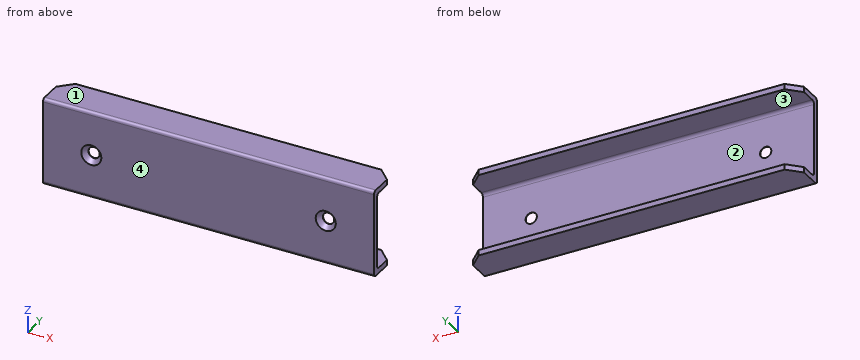
```python
from build123d import *

# Parameters (mm, degrees)
SKETCH1_W           = 105.55
SKETCH1_H           = 27.85
BOSS_EXTRUDE1_DEPTH = 11.5
SKETCH2_W           = 105.55
SKETCH2_H           = 24.35
CUT_EXTRUDE1_DEPTH  = 9.75
CHAMFER1_SIZE       = 4
FILLET1_R           = 1
HOLE1_D             = 3.6
HOLE1_CSINK_D       = 6.4
HOLE1_CSINK_ANGLE   = 82


with BuildPart() as part:
    # Sketch1 → Boss-Extrude1 (new body)
    with BuildSketch(Plane(origin=(0, 0, 0), x_dir=(1, 0, 0), z_dir=(0, 1, 0))):
        Rectangle(SKETCH1_W, SKETCH1_H)
    extrude(amount=BOSS_EXTRUDE1_DEPTH)

    # Sketch2 → Cut-Extrude1 (cut)
    with BuildSketch(Plane(origin=(0, 11.5, 0), x_dir=(1, 0, 0), z_dir=(0, 1, 0))):
        Rectangle(SKETCH2_W, SKETCH2_H)
    extrude(amount=-CUT_EXTRUDE1_DEPTH, mode=Mode.SUBTRACT)

    # Chamfer1
    chamfer1_edges = [part.edges().sort_by_distance(p)[0] for p in [
        (-52.775, 11.5, -13.05),
        (52.775, 11.5, -13.05),
        (-52.775, 11.5, 13.05),
        (52.775, 11.5, 13.05),
    ]]
    chamfer(chamfer1_edges, length=CHAMFER1_SIZE)

    # Fillet1
    fillet1_edges = [part.edges().sort_by_distance(p)[0] for p in [
        (0, 1.75, -12.175),
        (0, 1.75, 12.175),
        (0, 0, 13.925),
        (0, 0, -13.925),
    ]]
    fillet(fillet1_edges, radius=FILLET1_R)

    # Hole1 (through all)
    with Locations(Plane(origin=(-37.375, 0, 0), x_dir=(0, 0, -1), z_dir=(0, -1, 0))):
        with Locations((0, 0), (0, 74.75)):
            CounterSinkHole(HOLE1_D / 2, HOLE1_CSINK_D / 2, counter_sink_angle=HOLE1_CSINK_ANGLE)


solid = part.part
```
CAD build for the part. Positions are in the model's coordinates, mm. Face numbers are marked on the shaded views. Coordinates: 2 decimals unless noted, no trailing zeros. Order: outer loops, then holes, each group sorted by start corner. A loop starts at its lowest first (then second) coordinate and runs counter-clockwise, first axis right, second up. Notation, with made-up numbers: (86, 12) -> (129, 12) arc R25 ccw to (129, 24) -> close; hole circle Ø6 at (20.5, -4). An arc over 180 degrees is marked (long way). Use one line per item in the form item = value. Start each with the question number.
1) Band-saw the part on A-A on y = 4.5. Give the cut face in (x, z) (3 decimals), then the cut area to 3 significant figures.
2) Pull direction Z, two halves, no side cores. Call the marked faces 1, 2, 3 and 4: +Z half, -Z half, draft (parallel to the pull), parting line (faces both ways), or undercut.
3) Band-saw the part on C-C on x = -9.5. Give the cut face in (y, z) (3 decimals), then the cut area to 3 significant figures.
4) Band-saw the part on B-B on z = 0. Give the cut face in (x, y) (3 decimals).
5) Band-saw the part on D-D on z = -9.75. Give the cut face in (x, y) (3 decimals), then the cut area to 3 significant figures.
6) Drop flat-ended pins along their axis: pin 1 (4 mm diameter, centred on x = -37.375, z = 0, fed in from +Y); pin 2 (4.5 mm diameter, centred on x = 37.375, z = 0, fed in from -Y); pin 3 (6 mm diameter, centred on x = -15, z = 9, fed in from +Y). Give the stop position or say it passes through.
7) Drill centre lines: L1, parallel to X at y = 1.7, z = 0 (3 decimals); L2, parallel to Z at x = 46.5, y = 11 (3 decimals); L3, parallel to Y at x = -15, z = -4. Where is each one in solid material? Low to high. Write a range as [from, to].
Entries:
q1.outline = (-52.775, -13.925) -> (52.775, -13.925) -> (52.775, -12.175) -> (-52.775, -12.175) -> close; (-52.775, 12.175) -> (52.775, 12.175) -> (52.775, 13.925) -> (-52.775, 13.925) -> close
q1.area = 369 mm2
q2.face_1 = +Z half
q2.face_2 = undercut
q2.face_3 = undercut
q2.face_4 = draft
q3.outline = (0, -12.925) arc R1 ccw to (1, -13.925) -> (11.5, -13.925) -> (11.5, -12.175) -> (2.75, -12.175) arc R1 cw to (1.75, -11.175) -> (1.75, 11.175) arc R1 cw to (2.75, 12.175) -> (11.5, 12.175) -> (11.5, 13.925) -> (1, 13.925) arc R1 ccw to (0, 12.925) -> close
q3.area = 82.9 mm2
q4.outline = (-52.775, 0) -> (-40.575, 0) -> (-39.175, 1.611) -> (-39.175, 1.75) -> (-52.775, 1.75) -> close; (-35.575, 1.611) -> (-34.175, 0) -> (34.175, 0) -> (35.575, 1.611) -> (35.575, 1.75) -> (-35.575, 1.75) -> close; (39.175, 1.611) -> (40.575, 0) -> (52.775, 0) -> (52.775, 1.75) -> (39.175, 1.75) -> close
q5.outline = (-52.775, 0) -> (52.775, 0) -> (52.775, 1.75) -> (-52.775, 1.75) -> close
q5.area = 185 mm2
q6.pin_1 = 1.75
q6.pin_2 = 1.09
q6.pin_3 = 2.18
q7.L1 = [-52.775, -39.175], [-35.575, 35.575], [39.175, 52.775]
q7.L2 = [-13.925, -12.175], [12.175, 13.925]
q7.L3 = [0, 1.75]
